from build123d import *

# Parameters (mm, degrees)
SKETCH1_R           = 12.7
EXTRUDE1_DEPTH      = 152.4
CHAMFER1_SIZE       = 1.905
SKETCH3_W           = 6.35
SKETCH3_H           = 3.175
EXTRUDE2_DEPTH      = 153.4
EXTRUDE2_DEPTH_BACK = 153.4


with BuildPart() as part:
    # Sketch1 → Extrude1 (new body, symmetric)
    with BuildSketch(Plane(origin=(0, 0, 0), x_dir=(0, 0, -1), z_dir=(1, 0, 0))):
        Circle(SKETCH1_R)
    extrude(amount=EXTRUDE1_DEPTH, both=True)

    # Chamfer1
    chamfer1_edges = [part.edges().sort_by_distance(p)[0] for p in [
        (-152.4, 0, 12.7),
        (152.4, 0, 12.7),
    ]]
    chamfer(chamfer1_edges, length=CHAMFER1_SIZE)

    # Sketch3 → Extrude2 (cut, two sides)
    with BuildSketch(Plane(origin=(0, 0, 0), x_dir=(0, 0, -1), z_dir=(1, 0, 0))) as extrude2_sk:
        with Locations((0, 11.1125)):
            Rectangle(SKETCH3_W, SKETCH3_H)
    extrude(amount=EXTRUDE2_DEPTH, mode=Mode.SUBTRACT)
    extrude(extrude2_sk.sketch, amount=-EXTRUDE2_DEPTH_BACK, mode=Mode.SUBTRACT)


solid = part.part
Can you work these out from the model? Positions are in its coordinate system, mm. Coordinates: 2 decimals unless noted, no trailing zeros. Write each loop counter-clockwise with the first axis right and the second up, starting at its lowest first coordinate (ties: lowest second). Pieces come first, ordered by that corner, then holes. Notation, with made-up numbers: (-9, 34.25) - (26, 34.25) arc R33 cw to (26, 72.25) - close; hole circle Ø7 at (32, 44.5). An arc over 180 degrees is marked (long way). Return JSON: item names as keys, results as strings. Group by question number.
Item 1: We'd pull the mould along Z, two halves only. Please class faces 1 (the face through (-152.096, -11.09, 0.449)), 2 (the face through (-152.4, 0, 0)), 3 (the face through (-2, 9.525, 0)): pulls with the +Z half, pulls with the -Z half, needs draft (parallel to the pull), parting line crosses it, or undercut.
Item 2: If we section it at A-A (z = 0): Write out the boundary of the cut face in (x, y) (3 decimals), then the cut area to 3 significant figures.
Item 3: Please list where these lines run through material, in increasing order: probe 1 along Y at (x, z) = (-80, -0.5) (3 decimals); probe 2 along Z at (x, y) = (140.5, -6.75); probe 3 along Z at (x, y) = (-59, -1.5).
Item 4: I'm going to push flat-ended pins straight in: pin 1 Ø1.9 at (x, z) = (44, 0.5) entering from +Y (3 decimals); pin 2 Ø3 at (x, y) = (-88, -5) entering from +Z; pin 3 Ø10 at (x, z) = (-73.5, -8) entering from -Y. Where does each tip first touch, or does it pass through?
Item 5: If we section it at B-B (x = 2.5): Write out the boundary of the cut face in (y, z) (3 decimals), then the cut area to 3 significant figures.
Return value:
{
 "1": {"face 1": "parting line crosses it", "face 2": "needs draft", "face 3": "undercut"},
 "2": {"outline": "(-152.4, -10.795) - (-150.495, -12.7) - (150.495, -12.7) - (152.4, -10.795) - (152.4, 9.525) - (-152.4, 9.525) - close", "area": "6,770 mm^2"},
 "3": {"probe 1": "y = -12.69 to 9.525", "probe 2": "z = -10.76 to 10.76", "probe 3": "z = -12.61 to 12.61"},
 "4": {"pin 1": "stops at y = 9.525", "pin 2": "stops at z = 12.21", "pin 3": "stops at y = -12.34"},
 "5": {"outline": "(9.525, -3.175) - (9.525, 3.175) - (12.297, 3.175) arc R12.7 ccw (long way) to (12.297, -3.175) - close", "area": "487 mm^2"}
}
